from build123d import *

# Parameters (mm, degrees)
BOSS_EXTRUDE1_DEPTH = 39.6875
CUT_EXTRUDE1_DEPTH  = 12.7
CUT_EXTRUDE2_DEPTH  = 12.7
CUT_EXTRUDE3_DEPTH  = 3.175
CUT_EXTRUDE4_START  = -9.525
CUT_EXTRUDE4_DEPTH  = 3.175
CUT_EXTRUDE5_DEPTH  = 50.609375


with BuildPart() as part:
    # Sketch1 → Boss-Extrude1 (new body)
    with BuildSketch(Plane(origin=(0, 0, 0), x_dir=(1, 0, 0), z_dir=(0, 1, 0))):
        with BuildLine():
            Line((-12.7, 0), (-69.85, 0))
            Line((-69.85, 0), (-69.85, 25.4))
            Line((-69.85, 25.4), (-1.678775343, 25.4))
            Line((-1.678775343, 25.4), (19.05, 3.238927777))
            Line((19.05, 3.238927777), (19.05, -17.859375))
            ThreePointArc((19.05, -17.859375), (15.031784758, -23.765751202), (8.062510285, -22.19713815))
            Line((8.062510285, -22.19713815), (-12.7, 0))
        make_face()
    extrude(amount=BOSS_EXTRUDE1_DEPTH)

    # Sketch2 → Cut-Extrude1 (cut)
    with BuildSketch(Plane(origin=(0, 36.5125, 0), x_dir=(1, 0, 0), z_dir=(0, 1, 0))):
        with BuildLine():
            Line((12.7, -11.509375), (-1.934489816, -11.509375))
            Line((-1.934489816, -11.509375), (8.062510285, -22.19713815))
            ThreePointArc((8.062510285, -22.19713815), (18.525259479, -20.386992851), (12.7, -11.509375))
        make_face()
    extrude(amount=-CUT_EXTRUDE1_DEPTH, mode=Mode.SUBTRACT)

    # Sketch3 → Cut-Extrude2 (cut)
    with BuildSketch(Plane(origin=(0, 14.2875, 0), x_dir=(1, 0, 0), z_dir=(0, 1, 0))):
        with BuildLine():
            Line((12.7, -11.509375), (-1.934489816, -11.509375))
            Line((-1.934489816, -11.509375), (8.062510285, -22.19713815))
            ThreePointArc((8.062510285, -22.19713815), (18.525259479, -20.386992851), (12.7, -11.509375))
        make_face()
    extrude(amount=-CUT_EXTRUDE2_DEPTH, mode=Mode.SUBTRACT)

    # Sketch4 → Cut-Extrude3 (cut)
    with BuildSketch(Plane(origin=(0, 23.8125, 0), x_dir=(1, 0, 0), z_dir=(0, 1, 0))):
        with BuildLine():
            Line((12.7, -11.509375), (-1.934489816, -11.509375))
            Line((-1.934489816, -11.509375), (8.062510285, -22.19713815))
            ThreePointArc((8.062510285, -22.19713815), (6.874740521, -15.331757149), (12.7, -11.509375))
        make_face()
    extrude(amount=-CUT_EXTRUDE3_DEPTH, mode=Mode.SUBTRACT)

    # Sketch4<2> → Cut-Extrude4 (cut)
    with BuildSketch(Plane(origin=(0, 23.8125, 0), x_dir=(1, 0, 0), z_dir=(0, 1, 0)).offset(CUT_EXTRUDE4_START)):
        with BuildLine():
            Line((12.7, -11.509375), (-1.934489816, -11.509375))
            Line((-1.934489816, -11.509375), (8.062510285, -22.19713815))
            ThreePointArc((8.062510285, -22.19713815), (6.874740521, -15.331757149), (12.7, -11.509375))
        make_face()
    extrude(amount=CUT_EXTRUDE4_DEPTH, mode=Mode.SUBTRACT)

    # Sketch5 → Cut-Extrude5 (cut, through all)
    with BuildSketch(Plane(origin=(0, 0, -25.4), x_dir=(-1, 0, 0), z_dir=(0, 0, -1))):
        Polygon((69.85, 6.35), (12.7, 39.6875), (69.85, 39.6875), align=None)
    extrude(amount=-CUT_EXTRUDE5_DEPTH, mode=Mode.SUBTRACT)


solid = part.part
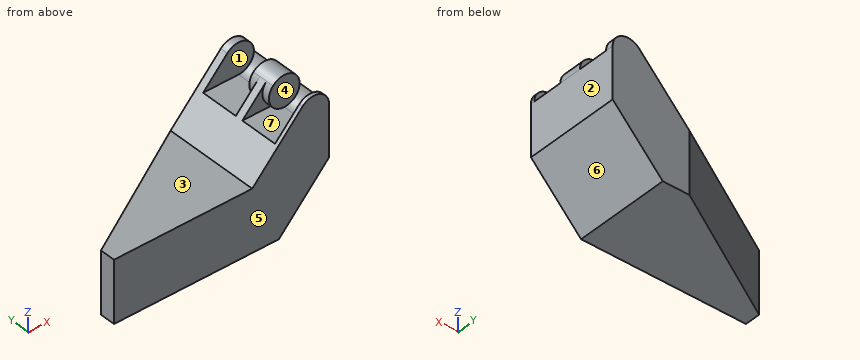
Here's how the part is built. I have some questions about the finished solid (model axes, mm). Face numbers are marked on the shaded views. A direction names the side the tool comes from. Give positions to 0.01 mm unless a question says otherwise; leave off trailing zeros. Order: outer loops, then holes, each group sorted by start corner. A loop starts at its lowest first (then second) coordinate and runs counter-clockwise, first axis right, second up. Notation, with made-up numbers: M -15,80.25 L 33,80.25 A14 ccw 33,101.25 Z; hole C 39,6 d3. An arc over 180 degrees is marked long. Answer as a JSON object with one key per item and string values. Group by question number.
1) Suppose I cut it at D-D, the plane y = 11.5. Write out the boundary of the cut face in (x, z), plus the area to 3 significant figures.
2) Suppose I cut it at C-C, the plane z = -22. Write out the boundary of the cut face in (x, y).
3) Suppose I cut it at B-B, the plane x = 3.5. Write out the boundary of the cut face in (y, z), plus the area to 3 significant figures.
4) Please list where these lines run through material, in increasing order: L1, parallel to Y at x = 8, z = 20; L2, parallel to Y at x = -61, z = -3; L3, parallel to Z at x = -25, y = 31.5. Write a range as [from, to].
5) Suppose I cut it at A-A, the plane y = 33.5. Write out the boundary of the cut face in (x, z), plus the area to 3 significant figures.
6) We'd pull the mould along Y, two halves only. Please class the marked faces 4, 5, 6 and 7: pulls with the +Y half, pulls with the -Y half, needs draft (parallel to the pull), parting line crosses it, or undercut.
7) On a 3-axis mill with a long thin cutter (end or side, diameter ignored), from which of +Z, -Z, +X, -X, +Y, -Y can I reach the whole of each face in a straight line? I mean the marked faces 1, 2 and 3. Say none if no direction works.
8) I'm going to push flat-ended pins straight in: pin 1 Ø12 at (x, y) = (-35.5, 8) entering from +Z; pin 2 Ø4 at (x, z) = (12.5, 17) entering from -Y; pin 3 Ø10 at (x, z) = (-35, -3.5) entering from +Y; pin 4 Ø11.5 at (x, y) = (2.5, 30.5) entering from +Z. Where does each tip first touch, or does it pass through?
Results found:
{
 "1": {"outline": "M -61.02,-25.4 L -1.68,-25.4 L 19.05,-3.24 L 19.05,17.86 A6.35 cw 12.7,11.51 L -1.93,11.51 L -12.7,0 L -61.02,0 Z", "area": "2,120 mm²"},
 "2": {"outline": "M -69.85,0 L 1.5,0 L 1.5,39.69 L -12.7,39.69 L -69.85,6.35 Z"},
 "3": {"outline": "M 0,-19.86 L 39.69,-19.86 L 39.69,17.32 L 36.51,17.32 L 36.51,11.51 L 20.64,11.51 L 20.64,17.32 L 17.46,17.32 L 17.46,11.51 L 1.59,11.51 L 1.59,17.32 L 0,17.32 Z", "area": "1,290 mm²"},
 "4": {"L1": "[0, 1.59], [14.29, 23.81], [36.51, 39.69]", "L2": "[0, 11.51]", "L3": "[-25.4, 0]"},
 "5": {"outline": "M -23.31,-25.4 L -1.68,-25.4 L 19.05,-3.24 L 19.05,17.86 A6.35 cw 12.7,11.51 L -1.93,11.51 L -12.7,0 L -23.31,0 Z", "area": "1,160 mm²"},
 "6": {"face 4": "undercut", "face 5": "pulls with the -Y half", "face 6": "needs draft", "face 7": "undercut"},
 "7": {"face 1": "+Z, -X", "face 2": "+Z, -Z, +X, +Y, -Y", "face 3": "+Z, -X, +Y, -Y"},
 "8": {"pin 1": "z = 0", "pin 2": "y = 0", "pin 3": "y = 29.6", "pin 4": "z = 11.51"}
}
